```python
from build123d import *

# Parameters (mm, degrees)
SKETCH36_R              = 0.6
SIDE_HOLES_DEPTH        = 2
CIRPATTERN2_COUNT       = 2
SKETCH37_R              = 35
SKETCH37_R_2            = 32.86364447
BOSS_EXTRUDE1_DEPTH     = 2
CHAMFER2_SIZE           = 1.75
CUT_EXTRUDE1_DEPTH      = 59.348970142
CUT_EXTRUDE1_DEPTH_BACK = 59.348970142


with BuildPart() as part:
    # Sketch35 → Revolve1 (revolve)
    with BuildSketch(Plane.XY, mode=Mode.PRIVATE) as revolve1_sk:
        Polygon((32.86364447, 28.896639018), (12.63, 0), (14.76635553, 0), (35, 28.896639018), align=None)
    revolve(revolve1_sk.sketch.rotate(Axis((0, 28.896639018, 0), (0, -1, 0)), 90), axis=Axis((0, 28.896639018, 0), (0, -1, 0)))

    # Sketch36 → side-holes (cut, symmetric)
    with BuildSketch(Plane(origin=(8.474857205, -5.9341589, 0), x_dir=(0, 0, 1), z_dir=(-0.8191520442889934, 0.5735764363510439, 0))):
        with Locations(Location((0, 18.744270391, 0), (0, 0, 235.340174101))):
            Circle(SKETCH36_R)
    side_holes = extrude(amount=SIDE_HOLES_DEPTH, both=True, mode=Mode.SUBTRACT)

    # CirPattern2: side-holes ×2 about axis
    cirpattern2_axis = Axis((0, 0, 0), (0, 1, 0))
    for i in range(1, CIRPATTERN2_COUNT):
        add(side_holes.rotate(cirpattern2_axis, i * 360 / CIRPATTERN2_COUNT), mode=Mode.SUBTRACT)

    # Sketch37 → Boss-Extrude1 (add)
    with BuildSketch(Plane(origin=(0, 28.896639018, 0), x_dir=(1, 0, 0), z_dir=(0, 1, 0))):
        with Locations(Location((0, 0, 0), (0, 0, 270))):
            Circle(SKETCH37_R)
        with Locations(Location((0, 0, 0), (0, 0, 270))):
            Circle(SKETCH37_R_2, mode=Mode.SUBTRACT)
    extrude(amount=BOSS_EXTRUDE1_DEPTH)

    # Chamfer2
    chamfer2_edges = [part.edges().sort_by_distance(p)[0] for p in [
        (0, 30.896639018, -35),
    ]]
    chamfer(chamfer2_edges, length=CHAMFER2_SIZE)

    # Sketch38 → Cut-Extrude1 (cut, two sides: drawn at the far end of the back side and taken through both)
    with BuildSketch(Plane.XY.offset(-CUT_EXTRUDE1_DEPTH_BACK)):
        with BuildLine():
            Line((-0.013961031, 28.260600049), (0, 28.246639018))
            Line((0, 28.246639018), (0.013961031, 28.260600049))
            ThreePointArc((0.013961031, 28.260600049), (2.93377117, 30.211554811), (6.377922061, 30.896639018))
            Line((6.377922061, 30.896639018), (-6.377922061, 30.896639018))
            ThreePointArc((-6.377922061, 30.896639018), (-2.93377117, 30.211554811), (-0.013961031, 28.260600049))
        make_face()
    extrude(amount=CUT_EXTRUDE1_DEPTH + CUT_EXTRUDE1_DEPTH_BACK, mode=Mode.SUBTRACT)


solid = part.part
```
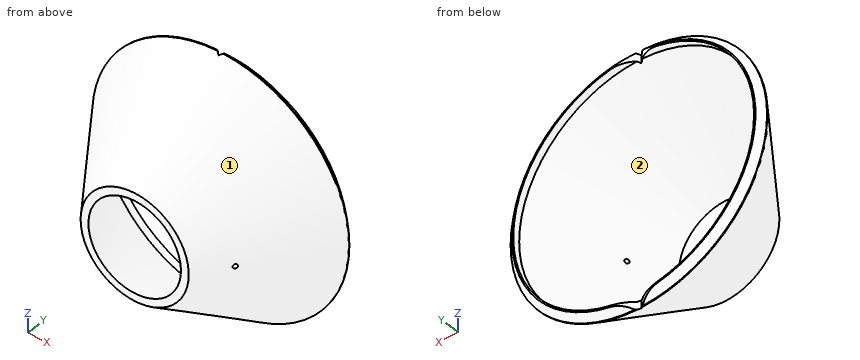
Could you check a few things on this model? Use its own coordinates, in mm. Face numbers are marked on the shaded views. Round coordinates to 2 decimals unless told otherwise and drop trailing zeros. Loops run counter-clockwise (first coordinate to the right, second up) from the corner with the lowest first, then second, coordinate; pieces in that order, holes last. Notation, with made-up numbers: (36.5, -9) - (71.5, -9) arc R18 ccw to (71.5, 25) - close; hole circle Ø4 at (84.25, 68). An arc over 180 degrees is marked (long way). Answer in a Markdown table with one row per item. Add a question column.
(1) If we section it at B-B (y = 5): Please give me the cut outline in (x, z), plus the area to 3 significant figures.
(2) I'm going to push flat-ended pins straight in: pin 1 (12 mm diameter, centred on x = -7.5, y = 6, fed in from -Z); pin 2 (4 mm diameter, centred on x = 12.5, y = 13.5, fed in from +Z); pin 3 (1.5 mm diameter, centred on x = 2.5, z = -28, fed in from -Y). Where does each tip first touch, or does it pass through?
(3) If we section it at A-A (y = 18.5): Please give me the cut outline in (x, z), plus the area to 3 significant figures.
(4) I need wall thicknesses on line 1 along Z through (x, y) = (17, 15); line 2 along X through (y, z) = (27.5, -28.5); line 3 along X through (y, z) = (16, -13). Which ranges of each line are inside material? Lowest first, please.
(5) If we mould it in two halves opening along Z, with no side actions, what happens to the marked faces 1 and 2? For each: pulls with the +Z half, pulls with the -Z half, needs draft (parallel to the pull), parting line crosses it, or undercut.
Model answer:
| question | item | result |
|---|---|---|
| 1 | outline | circle Ø36.53 at (0, 0); hole circle Ø32.26 at (0, 0) |
| 1 | area | 231 mm² |
| 2 | pin 1 | stops at z = -22.26 |
| 2 | pin 2 | stops at z = 22.69 |
| 2 | pin 3 | stops at y = 17.99 |
| 3 | outline | circle Ø55.44 at (0, 0); hole circle Ø51.17 at (0, 0) |
| 3 | area | 358 mm² |
| 4 | line 1 | z = -18.7 to -15.69, 15.69 to 18.7 |
| 4 | line 2 | x = -18.58 to -14.3, 14.3 to 18.58 |
| 4 | line 3 | x = -22.48 to -19.98, 19.98 to 22.48 |
| 5 | face 1 | parting line crosses it |
| 5 | face 2 | undercut |
